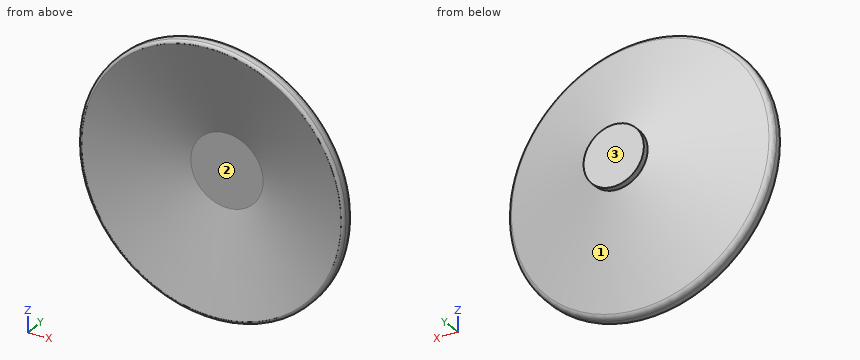
from build123d import *

# Parameters (mm, degrees)
FILLET1_R = 1
FILLET2_R = 0.5


with BuildPart() as part:
    # Sketch1 → Revolve1 (revolve)
    with BuildSketch(Plane.XY):
        Polygon((-6, 4.153212483), (-21.5, 0), (-22, 0), (-22, 2), (-5, 8.3), (-5, 9.3), (0, 9.3), (0, 4.153212483), align=None)
    revolve(axis=Axis((0, 57.053571429, 0), (0, -1, 0)))

    # Fillet1
    fillet1_edges = [part.edges().sort_by_distance(p)[0] for p in [
        (22, 2, 0),
    ]]
    fillet(fillet1_edges, radius=FILLET1_R)

    # Fillet2
    fillet2_edges = [part.edges().sort_by_distance(p)[0] for p in [
        (22, 0, 0),
    ]]
    fillet(fillet2_edges, radius=FILLET2_R - 0.0001)  # a hair under: the kernel refuses the full size


solid = part.part
Geometry check sheet. Reference: the model listing, model coordinates, mm. Face numbers are marked on the shaded views. Round coordinates to 2 decimals unless told otherwise and drop trailing zeros. Order: outer loops, then holes, each group sorted by start corner. A loop starts at its lowest first (then second) coordinate and runs counter-clockwise, first axis right, second up. Notation, with made-up numbers: M 88,-5 L 126,-5 A25 cw 126,30 Z; hole C -24,62 d8. An arc over 180 degrees is marked long. Answer in a Markdown table with one row per item.
(1) Go/stop test with flat-tipped pins: P1, Ø1.5, axis at x = -15.5, z = -8, coming from the +Y side; P2, Ø3, axis at x = 0.5, z = -13, coming from the +Y side; P3, Ø6, axis at x = -2.5, z = 0.5, coming from the -Y side. Record where each tip stops, or that it passes through.
Responses:
| item | result |
|---|---|
| P1 | stops at y = 3.97 |
| P2 | stops at y = 5.89 |
| P3 | stops at y = 4.15 |
(2) Sectioned sample at B-B, the plane y = 3.5. Record the cut outline in (x, z), and give its area (3 significant figures).
Responses:
| item | result |
|---|---|
| outline | C 0,0 d35.9; hole C 0,0 d16.88 |
| area | 789 mm² |
(3) Sectioned sample at A-A, the plane y = 7.75. Record the cut outline in (x, z), and give its area (3 significant figures).
Responses:
| item | result |
|---|---|
| outline | C 0,0 d12.97 |
| area | 132 mm² |
(4) Draft check along Z on the marked faces 1, 2 and 3. Enter one of: released by +Z, released by -Z, zero draft, split by the parting line, or undercut.
Responses:
| item | result |
|---|---|
| face 1 | split by the parting line |
| face 2 | undercut |
| face 3 | zero draft |
(5) Scan lines: probe 1 along Y at (x, z) = (6, -20); probe 2 along Y at (x, z) = (9.5, -5). Record each from-to range of solid material in increasing order. Write a range as from..to.
Responses:
| item | result |
|---|---|
| probe 1 | y = 0.17..2.41 |
| probe 2 | y = 2.88..6.17 |
